```python
from build123d import *

# Parameters (mm, degrees)
F1_DEPTH = 127
F3_DEPTH = 254
F7_DEPTH = 117.6922930425


with BuildPart() as f1:
    # F0 (on Front) → F1 (new body, symmetric)
    with BuildSketch(Plane.XZ):
        Polygon((0, 190.5), (0, 0), (254, 0), (254, 114.3), (127, 114.3), (127, 190.5), align=None)
    extrude(amount=F1_DEPTH, both=True)

    # F2 (on face) → F3 (cut)
    with BuildSketch(Plane.YZ.offset(127)):
        Polygon((127, 190.5), (0, 190.5), (127, 114.3), align=None)
    extrude(amount=-F3_DEPTH, mode=Mode.SUBTRACT)

    # F6 (on 3pt) → F7 (cut, through all)
    with BuildSketch(Plane(origin=(117.7900763359, -117.7900763359, 130.8778625954), x_dir=(0.8311676694, 0.3719590123, -0.4132877914), z_dir=(0.5560218569, -0.5560218569, 0.6178020632))):
        Polygon((163.877793469, -94.3983565734), (163.877793469, 76.4626688244), (11.0807048965, -17.9356877489), align=None)
    extrude(amount=F7_DEPTH, mode=Mode.SUBTRACT)


solid = f1.part
```
Read the model definition and answer for the solid it produces. Units are mm, in the model's axes. A direction names the side the tool comes from. Coordinates: 2 decimals unless noted, no trailing zeros. Write each loop counter-clockwise with the first axis right and the second up, starting at its lowest first coordinate (ties: lowest second). Pieces come first, ordered by that corner, then holes. Notation, with made-up numbers: (35.5, 82) -> (49.5, 82) arc R24 ccw to (49.5, 111) -> close; hole circle Ø6 at (22.5, 85.25). An arc over 180 degrees is marked (long way). Answer as a JSON object with one key per item and string values.
Q1. The part is cut by section D-D on y = 4. Give the vertices of the cut face in (x, z).
The answers:
{"outline": "(0, 0) -> (254, 0) -> (254, 114.3) -> (127, 114.3) -> (127, 188.1) -> (0, 188.1) -> close"}
Q2. A tool of negligible diameter and unlimited length cuts with its end or side. For faces 1 (the flat face through (127, -30, 152)), 2 (the flat face through (97, -127, 75)), from which of +Z, -Z, +X, -X, +Y, -Y can it reach the whole face along a straight path? Write none if from no direction.
The answers:
{"face 1": "+Z, +X, +Y, -Y", "face 2": "+Z, -Z, +X, -X, -Y"}
Q3. Flat-ended cylindrical pins translate along their axes: pin 1 Ø3 at (x, y) = (77.5, 36) entering from +Z; pin 2 Ø2 at (x, z) = (56, 133) entering from +Y; pin 3 Ø2 at (x, y) = (133.5, 19) entering from +Z; pin 4 Ø1 at (y, z) = (-86, 109.5) entering from -X. Find the tip coordinate at first contact, or state that the pin passes through.
The answers:
{"pin 1": "stops at z = 169.8", "pin 2": "stops at y = 97.5", "pin 3": "stops at z = 114.3", "pin 4": "stops at x = 0"}
Q4. Consider line 1 (Z direction, x = 195.5, y = 20.5); line 2 (Z direction, x = 38.5, y = 75); line 3 (X direction, y = -87, z = 160). Determine where each line is inside the solid, lowest interval first. Write a range as [from, to].
The answers:
{"line 1": "z = [0, 114.3]", "line 2": "z = [0, 145.5]", "line 3": "x = [0, 127]"}
Q5. The part is cut by section A-A on y = -50. Give the vertices of the cut face in (x, z), then the cut area to 3 significant figures.
The answers:
{"outline": "(0, 0) -> (254, 0) -> (254, 69.3) -> (204, 114.3) -> (127, 114.3) -> (127, 190.5) -> (0, 190.5) -> close", "area": "37,600 mm2"}
Q6. The part is cut by section C-C on z = 58.5. Give the vertices of the cut face in (x, y).
The answers:
{"outline": "(0, -127) -> (189, -127) -> (254, -62) -> (254, 127) -> (0, 127) -> close"}
Q7. The part is cut by section B-B on x = 55.5. Give the vertices of the cut face in (y, z).
The answers:
{"outline": "(-127, 0) -> (127, 0) -> (127, 114.3) -> (0, 190.5) -> (-127, 190.5) -> close"}
